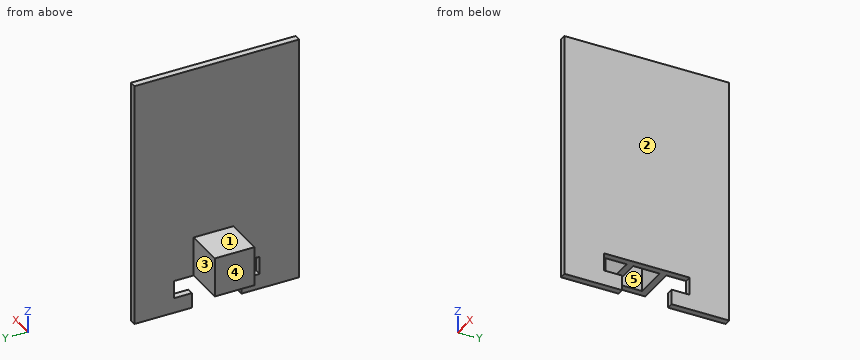
from build123d import *

# Parameters (mm, degrees)
SKETCH1_W           = 63.5
SKETCH1_H           = 95.25
BOSS_EXTRUDE1_DEPTH = 2.54
CUT_EXTRUDE1_DEPTH  = 13.97
SKETCH5_W           = 15.24
SKETCH5_H           = 15.24
BOSS_EXTRUDE2_DEPTH = 15.24
SKETCH6_W           = 12.7
SKETCH6_H           = 10.16
CUT_EXTRUDE2_DEPTH  = 12.7


with BuildPart() as part:
    # Sketch1 → Boss-Extrude1 (new body)
    with BuildSketch(Plane.YZ):
        with Locations((31.75, 47.625)):
            Rectangle(SKETCH1_W, SKETCH1_H)
    extrude(amount=BOSS_EXTRUDE1_DEPTH)

    # Sketch4 → Cut-Extrude1 (cut)
    with BuildSketch(Plane.YZ.offset(2.54)):
        Polygon((22.225, 0), (41.275, 0), (41.275, 5.842), (48.26, 5.842), (48.26, 12.7), (41.402, 12.7), (22.098, 12.7), (15.24, 12.7), (15.24, 5.842), (22.225, 5.842), align=None)
    extrude(amount=-CUT_EXTRUDE1_DEPTH, mode=Mode.SUBTRACT)

    # Sketch5 → Boss-Extrude2 (add)
    with BuildSketch(Plane(origin=(0, 0, 0), x_dir=(0, -1, 0), z_dir=(-1, 0, 0))):
        with Locations((-33.02, 20.32)):
            Rectangle(SKETCH5_W, SKETCH5_H)
    extrude(amount=BOSS_EXTRUDE2_DEPTH)

    # Sketch6 → Cut-Extrude2 (cut)
    with BuildSketch(Plane(origin=(0, 0, 12.7), x_dir=(1, 0, 0), z_dir=(0, 0, -1))):
        with Locations((-6.35, -33.02)):
            Rectangle(SKETCH6_W, SKETCH6_H)
    extrude(amount=-CUT_EXTRUDE2_DEPTH, mode=Mode.SUBTRACT)


solid = part.part
Check sheet for the modelled part. Datum: model origin and axes. Units: mm. Face numbers are marked on the shaded views. A direction names the side the tool comes from. Round coordinates to 2 decimals unless told otherwise and drop trailing zeros. Loops run counter-clockwise (first coordinate to the right, second up) from the corner with the lowest first, then second, coordinate; pieces in that order, holes last.
1. Set-up check for the marked faces 1 and 2: record each of +Z, -Z, +X, -X, +Y, -Y from which the full face is reachable in a straight line by a thin tool's end or side.
2. Scan lines: probe 1 along Y at (x, z) = (-5.75, 19); probe 2 along X at (y, z) = (30, 17.5); probe 3 along X at (y, z) = (22.5, 28.5). Record each from-to range of solid material in increasing order.
3. Mould release check, pull along Y, two halves, no side actions. Record for the marked faces 3, 4 and 5: released by +Y, released by -Y, zero draft, split by the parting line, or undercut.
4. Sectioned sample at B-B on x = -6.75. Record the boundary of the cut face in (y, z).
5. Gauge pin test, flat ends, axial feed: pin 1 Ø8 at (y, z) = (49.5, 85) entering from -X; pin 2 Ø4.5 at (x, z) = (-9, 20) entering from -Y; pin 3 Ø1.5 at (x, z) = (-10, 14.5) entering from +Y. Record the tip position at first contact, or that the pin passes through.
6. Sectioned sample at A-A on z = 16.5. Record the boundary of the cut face in (x, y).
7. Sectioned sample at C-C on y = 17.5. Record the boundary of the cut face in (x, z), and give its area (3 significant figures).
8. Sectioned sample at D-D on y = 29. Record the boundary of the cut face in (x, z).
Recorded:
1. face 1: +Z, -X, +Y, -Y
1. face 2: +Z, -Z, +X, +Y, -Y
2. probe 1: y = 25.4 to 27.94, 38.1 to 40.64
2. probe 2: x = -15.24 to -12.7, 0 to 2.54
2. probe 3: x = 0 to 2.54
3. face 3: released by +Y
3. face 4: zero draft
3. face 5: undercut
4. outline: (25.4, 12.7) - (27.94, 12.7) - (27.94, 25.4) - (38.1, 25.4) - (38.1, 12.7) - (40.64, 12.7) - (40.64, 27.94) - (25.4, 27.94) - close
5. pin 1: stops at x = 0
5. pin 2: stops at y = 25.4
5. pin 3: stops at y = 40.64
6. outline: (-15.24, 25.4) - (0, 25.4) - (0, 0) - (2.54, 0) - (2.54, 63.5) - (0, 63.5) - (0, 40.64) - (-15.24, 40.64) - close; hole (-12.7, 27.94) - (0, 27.94) - (0, 38.1) - (-12.7, 38.1) - close
7. outline: (0, 0) - (2.54, 0) - (2.54, 5.84) - (0, 5.84) - close; (0, 12.7) - (2.54, 12.7) - (2.54, 95.25) - (0, 95.25) - close
7. area: 225 mm2
8. outline: (-15.24, 12.7) - (-12.7, 12.7) - (-12.7, 25.4) - (0, 25.4) - (0, 12.7) - (2.54, 12.7) - (2.54, 95.25) - (0, 95.25) - (0, 27.94) - (-15.24, 27.94) - close
